Input: part model. Units: mm. Frame: model coordinates. Give positions to 0.01 mm unless a question says otherwise; leave off trailing zeros. Loops run counter-clockwise (first coordinate to the right, second up) from the corner with the lowest first, then second, coordinate; pieces in that order, holes last. Notation, with made-up numbers: (-10.5, -40) - (33.5, -40) arc R12 ccw to (33.5, -27) - close; hole circle Ø5 at (37, -22). An arc over 180 degrees is marked (long way). Answer as a JSON object with one key per item and string values. Group by question number.
(1) Material intervals for L1, parallel to Z at x = 568.5, y = 3.75; L2, parallel to Z at x = 502, y = 6; L3, parallel to X at y = 4.25, z = 1178, sorted ascending.
(2) Mould query, pull axis Z, two halves, no side actions, for faces 1 (the flat face through (188.598, 4.93, 356.253)), 2 (the flat face through (231, 0, 914)), 3 (the cylindrical face through (522.3, 4.93, 1042.11)), 4 (the flat face through (-153.62, 4.93, 745.75)). Classes: +Z half, -Z half, draft (parallel to the pull), parting line (faces both ways), or undercut.
(3) Pin query (flat end, axial travel): P1, Ø5, axis at x = 503, y = 5, coming from the -Z side. Return the tip coordinate at first contact, or that it passes through.
(4) Section query C-C (z = 260.5). Return loops of the section in (x, y).
(5) Section query D-D (x = 317). Return loops of the section in (y, z), plus the area to 3 significant figures.
(6) Section query A-A (z = 1228). Return loops of the section in (x, y).
(7) Section query B-B (x = 538.5). Return loops of the section in (y, z).
Solid Edge part; units mm, degrees
sketch "Sketch1" plane through (0, 0, 0) normal (0, -1, 0) x (1, 0, 0)
  line L0 (-73.0122, 1512.6678) -> (681.9878, 1512.6678)
  line L1 (681.9878, 1512.6678) -> (681.9878, 702.6678)
  line L2 (681.9878, 702.6678) -> (371.9878, 702.6678)
  line L3 (371.9878, 702.6678) -> (0, 0)
  line L4 (0, 0) -> (-232, 0)
  line L5 (-232, 0) -> (-73.0122, 1512.6678)
extrude "Protrusion1" add sketch "Sketch1" against normal blind 10
sketch "Sketch2" plane through (224.9939, 0, 756.3339) normal (0, -1, 0) x (1, 0, 0)
  circle A0 centre (301.9939, 655.0839) radius 36
  circle A1 centre (301.9939, 453.5781) radius 36
  circle A2 centre (301.9939, 250.0839) radius 36
  circle A3 centre (301.9939, 47.5839) radius 36
extrude "VaciadoExtruido_1" cut sketch "Sketch2" against normal blind 30.0194
sketch "Sketch3" plane through (-152.5061, 5, 756.3339) normal (-0.9945, 0, 0.1045) x (-0.1045, 0, -0.9945)
  circle A0 centre (-380.4677, 0) radius 3
extrude "VaciadoExtruido_2" cut sketch "Sketch3" against normal blind 10
sketch "Sketch4" plane through (-152.5061, 5, 756.3339) normal (-0.9945, 0, 0.1045) x (-0.1045, 0, -0.9945)
  circle A0 centre (368.3316, -0.0101) radius 3
extrude "VaciadoExtruido_3" cut sketch "Sketch4" against normal blind 10
Recorded:
{
 "1": {"L1": "z = 702.67 to 1512.67", "L2": "z = 702.67 to 778, 829.83 to 980.5, 1032.33 to 1184, 1235.83 to 1385.5, 1437.33 to 1512.67", "L3": "x = -108.19 to 510.33, 543.65 to 681.99"},
 "2": {"face 1": "-Z half", "face 2": "draft", "face 3": "undercut", "face 4": "+Z half"},
 "3": {"P1": "stops at z = 702.67"},
 "4": {"outline": "(-204.62, 0) - (137.91, 0) - (137.91, 10) - (-204.62, 10) - close"},
 "5": {"outline": "(0, 598.8) - (10, 598.8) - (10, 1512.67) - (0, 1512.67) - close", "area": "9,140 mm^2"},
 "6": {"outline": "(-102.93, 0) - (495.86, 0) - (495.86, 10) - (-102.93, 10) - close; (558.11, 0) - (681.99, 0) - (681.99, 10) - (558.11, 10) - close"},
 "7": {"outline": "(0, 702.67) - (10, 702.67) - (10, 769.81) - (0, 769.81) - close; (0, 838.03) - (10, 838.03) - (10, 972.31) - (0, 972.31) - close; (0, 1040.53) - (10, 1040.53) - (10, 1175.8) - (0, 1175.8) - close; (0, 1244.02) - (10, 1244.02) - (10, 1377.31) - (0, 1377.31) - close; (0, 1445.53) - (10, 1445.53) - (10, 1512.67) - (0, 1512.67) - close"}
}
